Verification items for the finished model (mm, model axes). A direction names the side the tool comes from. Coordinates: 2 decimals unless noted, no trailing zeros. Loops run counter-clockwise (first coordinate to the right, second up) from the corner with the lowest first, then second, coordinate; pieces in that order, holes last. Notation, with made-up numbers: (33.5, -24) - (90.5, -24) arc R18 cw to (90.5, 10) - close; hole circle Ø5 at (20, 74.25). An arc over 180 degrees is marked (long way). One line per item, written item: value. Start each with the question number.
(1) Section check A-A (y = 0). Record the boundary of the cut face in (x, z).
(2) Gauge pin test, flat ends, axial feed: P1, Ø2, axis at x = 6.5, z = 6, coming from the +Y side; P2, Ø3, axis at x = -7.5, y = -2, coming from the -Z side; P3, Ø12, axis at y = 10.5, z = 25, coming from the +X side. Record the tip position at first contact, or that the pin passes through.
(3) Thickness scan on probe 1 along Y at (x, z) = (0, 30.75); probe 2 along Y at (x, z) = (-0.5, 6); probe 3 along X at (y, z) = (3, 3.5). Record the ranges inside material, lowest first. Write a range as [from, to].
(4) Section check B-B (x = 0). Record the boundary of the cut face in (y, z).
(5) Draft check along X on faces 4 (the face through (-10.316, -7.91, 4.93)), 5 (the face through (4, -4, 40)), 6 (the face through (-13.887, -10.648, 19.72)). Enter one of: +X half, -X half, draft (parallel to the pull), parting line (faces both ways), or undercut.
(6) Set-up check for faces 1 (the face through (0.766, 10.385, 25.653)), 2 (the face through (14.296, 0.3, 4.93)), 3 (the face through (3, 13, 0)): record each of +Z, -Z, +X, -X, +Y, -Y from which the full face is reachable in a straight line by a thin tool's end or side.
(7) Section check D-D (z = 37). Record the boundary of the cut face in (x, y), plus the area to 3 significant figures.
(8) Section check C-C (x = 15). Record the boundary of the cut face in (y, z).
```python
from build123d import *

# Parameters (mm, degrees)
CROQUIS1_R              = 17.5
CROQUIS1_R_2            = 13
SALIENTE_EXTRUIR1_DEPTH = 10
CROQUIS2_R              = 17.5
SALIENTE_EXTRUIR2_DEPTH = 30
CROQUIS12_R             = 4
CORTAR_EXTRUIR1_DEPTH   = 48.037219306
CROQUIS13_R             = 1
CORTAR_EXTRUIR2_DEPTH   = 10
CROQUIS14_R             = 2
CORTAR_EXTRUIR3_DEPTH   = 48.037219306


with BuildPart() as part:
    # Croquis1 → Saliente-Extruir1 (new body)
    with BuildSketch(Plane.XY):
        Circle(CROQUIS1_R)
        Circle(CROQUIS1_R_2, mode=Mode.SUBTRACT)
    extrude(amount=SALIENTE_EXTRUIR1_DEPTH)

    # Croquis2 → Saliente-Extruir2 (add)
    with BuildSketch(Plane.XY.offset(10)):
        Circle(CROQUIS2_R)
    extrude(amount=SALIENTE_EXTRUIR2_DEPTH)

    # Croquis4 → Cortar-Revolución1 (revolve, cut)
    with BuildSketch(Plane(origin=(0, 0, 0), x_dir=(0, 0, -1), z_dir=(1, 0, 0)), mode=Mode.PRIVATE) as cortar_revoluci_n1_sk:
        Polygon((-10, 0), (-10, 13), (-15, 0), align=None)
    revolve(cortar_revoluci_n1_sk.sketch.rotate(Axis((0, 0, 40), (0, 0, -1)), 270), axis=Axis((0, 0, 40), (0, 0, -1)), mode=Mode.SUBTRACT)

    # Croquis12 → Cortar-Extruir1 (cut, through all)
    with BuildSketch(Plane.XY.offset(40)):
        Circle(CROQUIS12_R)
    extrude(amount=-CORTAR_EXTRUIR1_DEPTH, mode=Mode.SUBTRACT)

    # Croquis13 → Cortar-Extruir2 (cut)
    with BuildSketch(Plane(origin=(0, 0, 0), x_dir=(-1, 0, 0), z_dir=(0, 0, -1))):
        with Locations((-15.25, 0)):
            Circle(CROQUIS13_R)
        with Locations((15.25, 0)):
            Circle(CROQUIS13_R)
    extrude(amount=-CORTAR_EXTRUIR2_DEPTH, mode=Mode.SUBTRACT)

    # Croquis14 → Cortar-Extruir3 (cut, through all)
    with BuildSketch(Plane(origin=(0, 0, 0), x_dir=(1, 0, 0), z_dir=(0, 1, 0))):
        with Locations(Location((0, -27.5, 0), (0, 0, 90))):
            Circle(CROQUIS14_R)
    extrude(amount=CORTAR_EXTRUIR3_DEPTH, mode=Mode.SUBTRACT)


solid = part.part
```
Responses:
1. outline: (-17.5, 0) - (-16.25, 0) - (-16.25, 10) - (-14.25, 10) - (-14.25, 0) - (-13, 0) - (-13, 10) - (-4, 13.46) - (-4, 40) - (-17.5, 40) - close; (4, 13.46) - (13, 10) - (13, 0) - (14.25, 0) - (14.25, 10) - (16.25, 10) - (16.25, 0) - (17.5, 0) - (17.5, 40) - (4, 40) - close
2. P1: stops at y = 16.61
2. P2: stops at z = 11.44
2. P3: stops at x = 16.91
3. probe 1: y = [-17.5, -4], [4, 17.5]
3. probe 2: y = [-17.49, -12.99], [12.99, 17.49]
3. probe 3: x = [-17.24, -12.65], [12.65, 17.24]
4. outline: (-17.5, 0) - (-13, 0) - (-13, 10) - (-4, 13.46) - (-4, 40) - (-17.5, 40) - close; (4, 13.46) - (13, 10) - (13, 0) - (17.5, 0) - (17.5, 25.5) - (4, 25.5) - close; (4, 29.5) - (17.5, 29.5) - (17.5, 40) - (4, 40) - close
5. face 4: undercut
5. face 5: draft
5. face 6: parting line
6. face 1: +Y
6. face 2: -Z
6. face 3: -Z, +X, -X, +Y, -Y
7. outline: circle Ø35 at (0, 0); hole circle Ø8 at (0, 0)
7. area: 912 mm²
8. outline: (-9.01, 0) - (-0.97, 0) - (-0.97, 10) - (0.97, 10) - (0.97, 0) - (9.01, 0) - (9.01, 40) - (-9.01, 40) - close
